Input: part model. Units: mm. Frame: model coordinates. A direction names the side the tool comes from. Round coordinates to 2 decimals unless told otherwise and drop trailing zeros. Order: outer loops, then holes, each group sorted by start corner. A loop starts at its lowest first (then second) coordinate and runs counter-clockwise, first axis right, second up. Notation, with made-up numbers: (61, -1) -> (88, -1) arc R15 ccw to (88, 8) -> close; hole circle Ø7 at (-12, -21.5). An arc over 180 degrees is marked (long way). Use a Markdown table: item, result.
from build123d import *

# Parameters (mm, degrees)
SALIENTE_EXTRUIR1_DEPTH = 25
REDONDEO1_R             = 20
CORTAR_EXTRUIR1_DEPTH   = 10
CROQUIS3_W              = 70
CROQUIS3_H              = 15
CORTAR_EXTRUIR2_DEPTH   = 135.692464426


with BuildPart() as part:
    # Croquis1 → Saliente-Extruir1 (new, symmetric)
    with BuildSketch(Plane.XY):
        Polygon((0, 5), (0, 0), (-90, 0), (-90, 71.370702608), (-24.226182617, 102.04153736), (-20, 92.978459489), (-80, 65), (-80, 5), align=None)
    extrude(amount=SALIENTE_EXTRUIR1_DEPTH, both=True)

    # Redondeo1
    redondeo1_edges = [part.edges().sort_by_distance(p)[0] for p in [
        (-90, 71.370702608, 0),
        (-80, 65, 0),
    ]]
    fillet(redondeo1_edges, radius=REDONDEO1_R)

    # Croquis2 → Cortar-Extruir1 (cut)
    with BuildSketch(Plane(origin=(0, 5, 0), x_dir=(1, 0, 0), z_dir=(0, 1, 0))):
        Polygon((-80, 10), (-80, -10), (-10, -10), (0, -17.5), (0, 17.5), (-10, 10), align=None)
        Polygon((-10, 25), (0, 17.5), (0, 25), align=None)
        Polygon((0, -17.5), (-10, -25), (0, -25), align=None)
    extrude(amount=-CORTAR_EXTRUIR1_DEPTH, mode=Mode.SUBTRACT)

    # Croquis3 → Cortar-Extruir2 (cut, through all)
    with BuildSketch(Plane(origin=(0, 5, 0), x_dir=(1, 0, 0), z_dir=(0, 1, 0))):
        with Locations((-45, -17.5)):
            Rectangle(CROQUIS3_W, CROQUIS3_H)
        with Locations((-45, 17.5)):
            Rectangle(CROQUIS3_W, CROQUIS3_H)
    extrude(amount=CORTAR_EXTRUIR2_DEPTH, mode=Mode.SUBTRACT)


solid = part.part
1) Ray query, probe 1 along Z at (x, y) = (-30, 4); probe 2 along X at (y, z) = (41.5, 23); probe 3 along Y at (x, z) = (-51.5, -19). Return the intervals inside material, ascending.
Answer key:
| item | result |
|---|---|
| probe 1 | z = -25 to -10, 10 to 25 |
| probe 2 | x = -90 to -80 |
| probe 3 | y = 0 to 5 |
2) Cut plane A-A on x = -11.5. Return loops of the section in (y, z), and give its area (3 significant figures).
Answer key:
| item | result |
|---|---|
| outline | (0, -25) -> (5, -25) -> (5, -10) -> (0, -10) -> close; (0, 10) -> (5, 10) -> (5, 25) -> (0, 25) -> close |
| area | 150 mm^2 |
3) Contact query for flat-ended pins moving along their axis: P1, Ø25, axis at y = 25, z = 2, coming from the +X side; P2, Ø12, axis at x = -65, z = 14.5, coming from the +Y side; P3, Ø16.5, axis at x = -40.5, z = 15, coming from the +Y side. Output: stop coordinate, or through.
Answer key:
| item | result |
|---|---|
| P1 | stops at x = -80 |
| P2 | stops at y = 84.88 |
| P3 | stops at y = 97.51 |
4) Cut plane D-D on y = 47.5. Return loops of the section in (x, z).
Answer key:
| item | result |
|---|---|
| outline | (-90, -25) -> (-80, -25) -> (-80, 25) -> (-90, 25) -> close |
5) Draft query along Z for faces 1 (the face through (-4.93, 2.54, -13.8)), 2 (the face through (-82, 24, 25)), 3 (the face through (-41, 5, -17)). Return one class per face: released by +Z, released by -Z, zero draft, split by the parting line, or undercut.
Answer key:
| item | result |
|---|---|
| face 1 | undercut |
| face 2 | released by +Z |
| face 3 | zero draft |
6) Set-up query: faces 4 (the face through (-45, 3, -10)), 5 (the face through (-52, 83, 10)), 6 (the face through (-5.07, 2.54, 13.7)). Return all of +Z, -Z, +X, -X, +Y, -Y with unobstructed straight access to the full face (end or side cutting, diameter ignored); none if empty.
Answer key:
| item | result |
|---|---|
| face 4 | +X, -Y |
| face 5 | +Z, +X, +Y |
| face 6 | +X, +Y, -Y |
7) Cut plane B-B on z = -1.5. Return loops of the section in (x, y), and give its area (3 significant figures).
Answer key:
| item | result |
|---|---|
| outline | (-90, 0) -> (-80, 0) -> (-80, 52.26) arc R20 cw to (-68.45, 70.38) -> (-20, 92.98) -> (-24.23, 102.04) -> (-78.45, 76.76) arc R20 ccw to (-90, 58.63) -> close |
| area | 1,380 mm^2 |
8) Cut plane C-C on x = -72.5. Return loops of the section in (y, z).
Answer key:
| item | result |
|---|---|
| outline | (0, -25) -> (5, -25) -> (5, -10) -> (0, -10) -> close; (0, 10) -> (5, 10) -> (5, 25) -> (0, 25) -> close; (67.87, -10) -> (79.53, -10) -> (79.53, 10) -> (67.87, 10) -> close |
